For this review, use the dimensioned drawing (mm, ordinates from the lowest corner) and the shaded views. Round coordinates to 2 decimals unless told otherwise and drop trailing zeros. Write each loop counter-clockwise with the first axis right and the second up, starting at its lowest first coordinate (ties: lowest second). Pieces come first, ordered by that corner, then holes. Notation, with made-up numbers: M 48.25,4 L 62.25,4 A16 ccw 62.25,13 Z; hole C 55.5,-22.5 d6. An arc over 180 degrees is marked long. One line per question, with ' | ' between items. Start each with the question number.
Item 1: Insertion check: pin 1 Ø0.5 at (x, z) = (8, 8.5) entering from +Y; pin 2 Ø3 at (x, y) = (25, 40) entering from +Z; pin 3 Ø2.5 at (x, y) = (44, 33) entering from +Z. Each pin has a flat end and moves straight along its axis. Give the tip position at first contact, or say it passes through.
Item 2: Add section A-A, the plane x = 40. State the section outline as (y, z) points, and give its area (3 significant figures).
Item 3: For L1, parallel to Y at x = 43.5, z = 7.5; L2, parallel to Y at x = 11.5, z = 8.75; L3, parallel to Z at x = 46, y = 68.5, list the stretches that pass through material, from the lowest coordinate up.
Item 4: Add section B-B, the plane y = 71.5. State the section outline as (x, z) points, and give its area (3 significant figures).
Item 5: Add section D-D, the plane y = 22. State the section outline as (x, z) points, and give its area (3 significant figures).
Item 6: Draft analysis for pull direction Z (two halves, no side actions). For the marked faces 1 and 2, state which applies: released by +Z, released by -Z, zero draft, split by the parting line, or undercut.
Item 7: Add section C-C, the plane x = 49.5. State the section outline as (y, z) points, and give its area (3 significant figures).
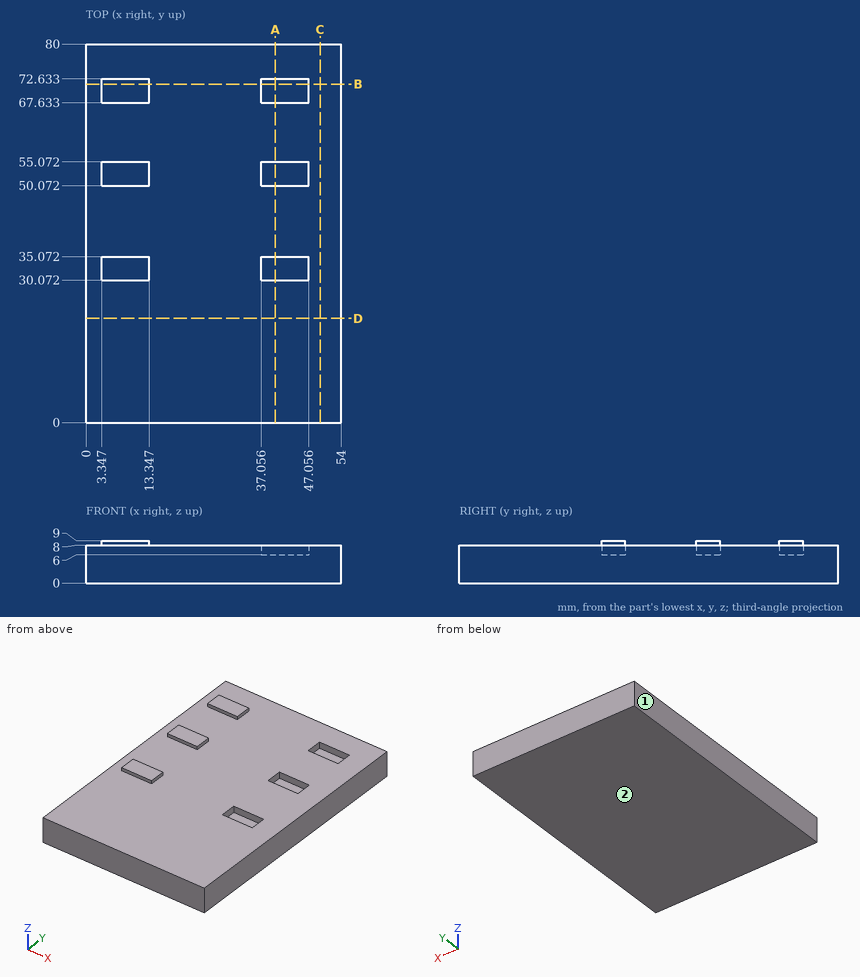
Computed values:
1) pin 1: stops at y = 72.63 | pin 2: stops at z = 8 | pin 3: stops at z = 6
2) outline: M 0,0 L 80,0 L 80,8 L 72.63,8 L 72.63,6 L 67.63,6 L 67.63,8 L 55.07,8 L 55.07,6 L 50.07,6 L 50.07,8 L 35.07,8 L 35.07,6 L 30.07,6 L 30.07,8 L 0,8 Z | area: 610 mm^2
3) L1: y = 0 to 30.07, 35.07 to 50.07, 55.07 to 67.63, 72.63 to 80 | L2: y = 30.07 to 35.07, 50.07 to 55.07, 67.63 to 72.63 | L3: z = 0 to 6
4) outline: M 0,0 L 54,0 L 54,8 L 47.06,8 L 47.06,6 L 37.06,6 L 37.06,8 L 13.35,8 L 13.35,9 L 3.35,9 L 3.35,8 L 0,8 Z | area: 422 mm^2
5) outline: M 0,0 L 54,0 L 54,8 L 0,8 Z | area: 432 mm^2
6) face 1: zero draft | face 2: released by -Z
7) outline: M 0,0 L 80,0 L 80,8 L 0,8 Z | area: 640 mm^2
